The listing builds one solid part. Answer for the finished solid, in the listing's coordinates (mm). A direction names the side the tool comes from. Coordinates: 2 decimals unless noted, no trailing zeros. Order: outer loops, then holes, each group sorted by start corner. A loop starts at its lowest first (then second) coordinate and runs counter-clockwise, first axis right, second up.
```python
from build123d import *

# Parameters (mm, degrees)
EXTRUDE_THIN1_DEPTH = 10
BOSS_EXTRUDE1_DEPTH = 2
BOSS_EXTRUDE2_START = -10
BOSS_EXTRUDE2_DEPTH = 2
SKETCH3_R           = 0.75
CUT_EXTRUDE1_DEPTH  = 56.66160031
BOSS_EXTRUDE3_START = -8
BOSS_EXTRUDE3_DEPTH = 4


with BuildPart() as part:
    # Sketch1 → Extrude-Thin1 (new body)
    with BuildSketch(Plane(origin=(-21.326839193, -3.611933395, 0), x_dir=(1, 0, 0), z_dir=(0, 0, 1))):
        Polygon((40.837274636, 20.62649088), (49.842183721, 10.115955591), (66.565347849, 6.191262572), (67.022304548, 8.13836056), (50.935628307, 11.913678763), (42.35608206, 21.927730293), align=None)
    extrude(amount=EXTRUDE_THIN1_DEPTH)

    # Sketch2 → Boss-Extrude1 (add)
    with BuildSketch(Plane.XY.offset(10)):
        Polygon((19.510435444, 17.014557485), (28.32605504, 24.567346264), (34.604051118, 17.239665473), (47.944334875, 14.108887223), (45.238508656, 2.579329178), (28.515344528, 6.504022197), align=None)
    extrude(amount=BOSS_EXTRUDE1_DEPTH)

    # Sketch2<2> → Boss-Extrude2 (add)
    with BuildSketch(Plane.XY.offset(10).offset(BOSS_EXTRUDE2_START)):
        Polygon((21.029242867, 18.315796898), (19.510435444, 17.014557485), (28.515344528, 6.504022197), (45.238508656, 2.579329178), (45.695465355, 4.526427166), (29.608789115, 8.301745368), align=None)
        Polygon((28.32605504, 24.567346264), (21.029242867, 18.315796898), (29.608789115, 8.301745368), (45.695465355, 4.526427166), (47.944334875, 14.108887223), (34.604051118, 17.239665473), align=None)
    extrude(amount=-BOSS_EXTRUDE2_DEPTH)

    # Sketch3 → Cut-Extrude1 (cut, through all)
    with BuildSketch(Plane.XY.offset(12)):
        with Locations((28.885341988, 7.156403894)):
            Circle(SKETCH3_R)
    extrude(amount=-CUT_EXTRUDE1_DEPTH, mode=Mode.SUBTRACT)

    # Sketch4 → Boss-Extrude3 (add)
    with BuildSketch(Plane.XY.offset(12).offset(BOSS_EXTRUDE3_START)):
        Polygon((26.37923513, 8.997290369), (25.447689261, 10.084591266), (21.423335505, 6.636723131), (21.434748512, -5.051368103), (20.008730224, -7.513493145), (23.089867331, -11.79022436), (24.164473573, -6.548039274), (22.365676805, -5.506208724), (22.354881373, 5.549422234), align=None)
    extrude(amount=BOSS_EXTRUDE3_DEPTH)


solid = part.part
```
(1) Find section B-B (z = 5.75). Write down the section's boundary in (x, y).
(2) The mould has two halves that part along X. Classify faces 6 (the face through (35, 12, 10)), 7 (the face through (29.32, 7.77, 5.1)), 8 (the face through (23.46, 8.38, 5.97)), 9 (the face through (25.38, 13.24, 4.93)): released by +X, released by -X, zero draft, split by the parting line, or undercut.
(3) Each of these flat-tipped pins is pushed along its axis until it touches: pin 1 Ø3 at (x, z) = (24, 3.5) entering from +Y; pin 2 Ø1.5 at (y, z) = (4.5, 3) entering from +X. Where does it stop, or does it pass through?
(4) Find section C-C (y = 20). Write down the section's boundary in (x, z), and give its area (3 significant figures).
(5) Find section D-D (y = 14.5). Write down the section's boundary in (x, z).
(6) Consider line 1 (Z direction, x = 28, y = 17.5); line 2 (Y direction, x = 28.75, z = 9.5); line 3 (Y direction, x = 30.5, z = -1). Determine where each line is inside the solid, lowest interval first.
(7) For faces 1 (the face through (22, -2, 8)), 2 (the face through (24.34, 7.25, 5.97)), 3 (the face through (22, -2, 4)), 4 (the face through (34, 15, 0)), 5 (the face through (23.278, -6.034, 5.972)), determine the directions among +Z, -Z, +X, -X, +Y, -Y from which every point of the face is accessible in a straight line to the end or side of a thin tool.
(8) Find section A-A (x = 25). Write down the section's boundary in (y, z), and give its area (3 significant figures).
Findings below:
1. outline: (19.51, 17.01) - (25.45, 10.08) - (21.42, 6.64) - (21.43, -5.05) - (20.01, -7.51) - (23.09, -11.79) - (24.16, -6.55) - (22.37, -5.51) - (22.35, 5.55) - (26.38, 9) - (28.18, 6.89) arc R0.75 cw (long way) to (28.93, 6.41) - (45.24, 2.58) - (45.7, 4.53) - (29.61, 8.3) - (21.03, 18.32) - close
2. face 6: zero draft
2. face 7: undercut
2. face 8: released by -X
2. face 9: released by +X
3. pin 1: stops at y = 16.6
3. pin 2: stops at x = 45.7
4. outline: (23, -2) - (32.24, -2) - (32.24, 0) - (23, 0) - close; (23, 10) - (32.24, 10) - (32.24, 12) - (23, 12) - close
4. area: 37.0 mm2
5. outline: (21.66, -2) - (46.28, -2) - (46.28, 0) - (24.3, 0) - (24.3, 10) - (46.28, 10) - (46.28, 12) - (21.66, 12) - close
6. line 1: z = -2 to 0, 10 to 12
6. line 2: y = 7.89 to 9.3
6. line 3: y = 6.04 to 22.03
7. face 1: +Z, -X, -Y
7. face 2: +Z, -Z
7. face 3: -Z, -X, -Y
7. face 4: +X, +Y
7. face 5: +Z, -Z, +X
8. outline: (7.82, 4) - (9.7, 4) - (9.7, 8) - (7.82, 8) - close; (10.61, -2) - (21.72, -2) - (21.72, 0) - (13.68, 0) - (13.68, 10) - (21.72, 10) - (21.72, 12) - (10.61, 12) - close
8. area: 82.7 mm2
